For this review, use the dimensioned drawing (mm, ordinates from the lowest corner) and the shaded views. A direction names the side the tool comes from. Give positions to 0.01 mm unless a question says otherwise; leave off trailing zeros. Write each loop counter-clockwise with the first axis right and the second up, starting at its lowest first coordinate (ties: lowest second). Pieces come first, ordered by that corner, then holes.
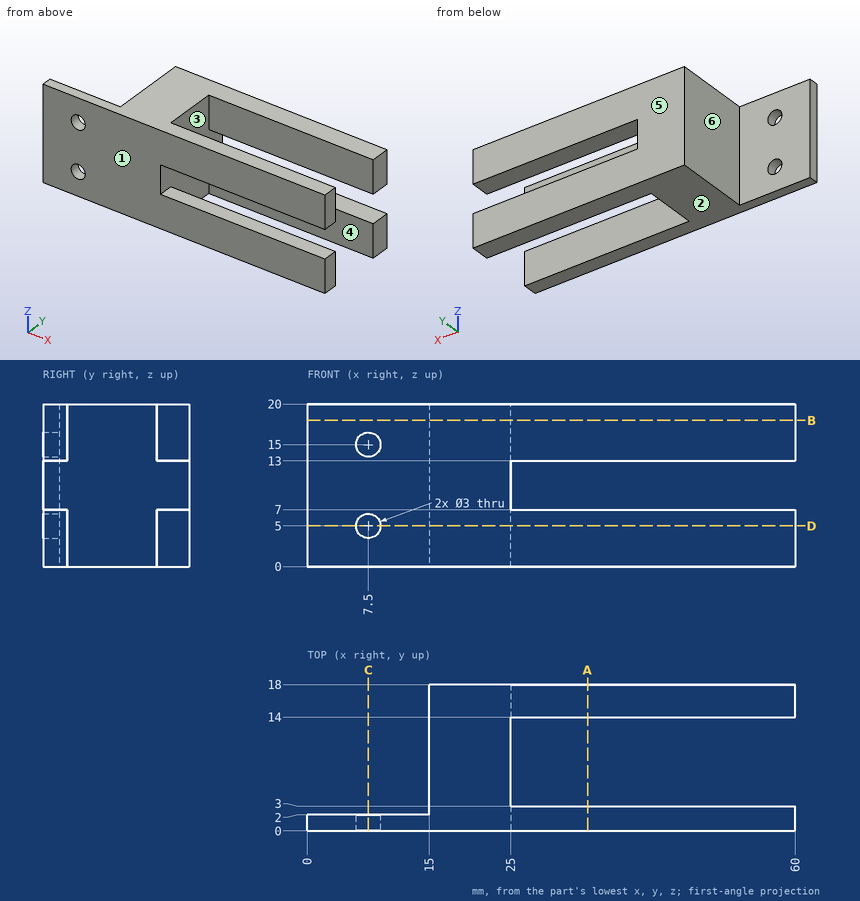
(1) We need section B-B (z = 18). Write out the cut boundary in (x, y), and give its area (3 significant figures).
(2) We need section A-A (x = 34.5). Write out the cut boundary in (y, z).
(3) Tool access review of the marked faces 4, 5 and 6: name each direction out of +Z, -Z, +X, -X, +Y, -Y from which nothing blocks a thin tool from reaching the whole face with its end or side.
(4) Clearance check with flat-ended pins moving along their axes: pin 1 Ø3 at (y, z) = (12, 10) entering from +X; pin 2 Ø8 at (y, z) = (11.5, 12) entering from -X; pin 3 Ø5 at (x, z) = (7.5, 15) entering from +Y. State where each tip first meets the part, or that it passes through.
(5) We need section C-C (x = 7.5). Write out the cut boundary in (y, z), and give its area (3 significant figures).
(6) The part is to be moulded in two halves that separate along Z. For the marked faces 1, 2 and 3, say which applies: +Z half, -Z half, draft (parallel to the pull), parting line (faces both ways), or undercut.
(7) For L1, parallel to Z at x = 7.5, y = 0.9; L2, parallel to Y at x = 44.5, z = 17.75; L3, parallel to X at y = 1.3, z = 15, list the stretches that pass through material, from the lowest coordinate up.
(8) We need section D-D (z = 5). Write out the cut boundary in (x, y).
The answers:
1. outline: (0, 0) - (60, 0) - (60, 3) - (25, 3) - (25, 14) - (60, 14) - (60, 18) - (15, 18) - (15, 2) - (0, 2) - close
1. area: 455 mm2
2. outline: (0, 0) - (3, 0) - (3, 7) - (0, 7) - close; (0, 13) - (3, 13) - (3, 20) - (0, 20) - close; (14, 0) - (18, 0) - (18, 7) - (14, 7) - close; (14, 13) - (18, 13) - (18, 20) - (14, 20) - close
3. face 4: +Z, -Z, +X
3. face 5: +Z, -Z, +X, -X, +Y
3. face 6: +Z, -Z, -X, +Y
4. pin 1: stops at x = 25
4. pin 2: stops at x = 15
4. pin 3: stops at y = 2
5. outline: (0, 0) - (2, 0) - (2, 3.5) - (0, 3.5) - close; (0, 6.5) - (2, 6.5) - (2, 13.5) - (0, 13.5) - close; (0, 16.5) - (2, 16.5) - (2, 20) - (0, 20) - close
5. area: 28.0 mm2
6. face 1: draft
6. face 2: -Z half
6. face 3: undercut
7. L1: z = 0 to 3.5, 6.5 to 13.5, 16.5 to 20
7. L2: y = 0 to 3, 14 to 18
7. L3: x = 0 to 6, 9 to 60
8. outline: (0, 0) - (6, 0) - (6, 2) - (0, 2) - close; (9, 0) - (60, 0) - (60, 3) - (25, 3) - (25, 14) - (60, 14) - (60, 18) - (15, 18) - (15, 2) - (9, 2) - close
